Could you check a few things on this model? Use its own coordinates, in mm. A direction names the side the tool comes from. Coordinates: 2 decimals unless noted, no trailing zeros. Loops run counter-clockwise (first coordinate to the right, second up) from the corner with the lowest first, then second, coordinate; pieces in that order, holes last. Notation, with made-up numbers: (75.5, 21) -> (112.5, 21) arc R19 cw to (112.5, 35) -> close; hole circle Ø7 at (-30.75, 69.25). An arc over 180 degrees is marked (long way). One line per question, with ' | ' between items.
```python
from build123d import *

# Parameters (mm, degrees)
SKETCH1_W            = 198
SKETCH1_H            = 256
SKETCH1_W_2          = 172.6
SKETCH1_H_2          = 230.6
MAINBODY_DEPTH       = 1.5875
M3_CLEARANCE_HOLE1_D = 3.6
INSIDEFILLET_R       = 10
FILLET2_R            = 5
M3_CLEARANCE_HOLE2_D = 3.6


with BuildPart() as part:
    # Sketch1 → MainBody (new body)
    with BuildSketch(Plane(origin=(0, 0, 0), x_dir=(1, 0, 0), z_dir=(0, 1, 0))):
        Rectangle(SKETCH1_W, SKETCH1_H)
        Rectangle(SKETCH1_W_2, SKETCH1_H_2, mode=Mode.SUBTRACT)
    extrude(amount=MAINBODY_DEPTH)

    # M3 Clearance Hole1 (through all)
    with Locations(Plane(origin=(0, 1.5875, 0), x_dir=(1, 0, 0), z_dir=(0, 1, 0))):
        with Locations((-92.65, 99), (-92.65, 29), (-92.65, -29), (-92.65, -99), (92.65, -99), (92.65, -29), (92.65, 29), (92.65, 99), (0, 121.65), (-49.5, 121.65), (49.5, -121.65), (0, -121.65), (-49.5, -121.65), (49.5, 121.65)):
            Hole(M3_CLEARANCE_HOLE1_D / 2)

    # InsideFillet
    insidefillet_edges = [part.edges().sort_by_distance(p)[0] for p in [
        (86.3, 0.79375, 115.3),
        (86.3, 0.79375, -115.3),
        (-86.3, 0.79375, -115.3),
        (-86.3, 0.79375, 115.3),
    ]]
    fillet(insidefillet_edges, radius=INSIDEFILLET_R)

    # Fillet2
    fillet2_edges = [part.edges().sort_by_distance(p)[0] for p in [
        (99, 0.79375, 128),
        (-99, 0.79375, 128),
        (-99, 0.79375, -128),
        (99, 0.79375, -128),
    ]]
    fillet(fillet2_edges, radius=FILLET2_R)

    # M3 Clearance Hole2 (through all)
    with Locations(Plane(origin=(0, 1.5875, 0), x_dir=(1, 0, 0), z_dir=(0, 1, 0))):
        with Locations((-81.072343025, 123), (106.927656975, 123), (94, -122.975), (-99.732934362, -43.278306391)):
            Hole(M3_CLEARANCE_HOLE2_D / 2)


solid = part.part
```
Q1. For faces 1 (the face through (-88, 1.588, -1)), 2 (the face through (-83.29, 0.8, 112.45)), which set-ups out of +Z, -Z, +X, -X, +Y, -Y let a thin tool reach every point of the face, with its end or its side?
Values follow:
face 1: +Z, -Z, +X, -X, +Y | face 2: +Y, -Y
Q2. Imagine slicing it at B-B on z = 19. Write out the boundary of the cut face in (x, y), plus the area to 3 significant figures.
Values follow:
outline: (-99, 0) -> (-86.3, 0) -> (-86.3, 1.59) -> (-99, 1.59) -> close; (86.3, 0) -> (99, 0) -> (99, 1.59) -> (86.3, 1.59) -> close | area: 40.3 mm2
Q3. For pin 1 (3 mm diameter, centred on x = 49.5, z = -121.65, fed in from +Y), with a flat end and sliding along its axis, tell me the tip position at first contact or that it passes through.
Values follow:
pin 1: passes through
Q4. Please list where these lines run through material, in increasing order: L1, parallel to Z at x = 49.5, y = 1.2; L2, parallel to X at y = 0.65, z = -29; L3, parallel to Z at x = 26, y = 1.55. Write a range as [from, to].
Values follow:
L1: z = [-128, -123.45], [-119.85, -115.3], [115.3, 119.85], [123.45, 128] | L2: x = [-99, -94.45], [-90.85, -86.3], [86.3, 90.85], [94.45, 99] | L3: z = [-128, -115.3], [115.3, 128]
Q5. We'd pull the mould along Z, two halves only. Please class faces 3 (the face through (97, 1, -127)), 4 (the face through (-98, 1, 126)), 5 (the face through (-83.45, 0.8, -112.29)), 6 (the face through (-88, 0, -1)): released by +Z, released by -Z, zero draft, split by the parting line, or undercut.
Values follow:
face 3: released by -Z | face 4: released by +Z | face 5: undercut | face 6: zero draft
Q6. Imagine slicing it at C-C on y = 0.95. Give the number of separate pieces and of enclosed holes in the cut face, plus the area to 3 significant figures.
Values follow:
separate pieces: 1 | enclosed holes: 17 | area: 10,800 mm2
Q7. Imagine slicing it at A-A on x = -66.5. Write out the boundary of the cut face in (y, z).
Values follow:
outline: (0, -128) -> (1.59, -128) -> (1.59, -115.3) -> (0, -115.3) -> close; (0, 115.3) -> (1.59, 115.3) -> (1.59, 128) -> (0, 128) -> close
